Check sheet for the modelled part. Datum: model origin and axes. Units: mm. A direction names the side the tool comes from. Give positions to 0.01 mm unless a question says otherwise; leave off trailing zeros. Loops run counter-clockwise (first coordinate to the right, second up) from the corner with the lowest first, then second, coordinate; pieces in that order, holes last. Notation, with made-up numbers: M 66.5,13 L 79.5,13 A33 cw 79.5,50 Z; hole C -20.5,25.25 d6. An arc over 180 degrees is marked long. Put each result on its own line as item: value. Start each with the question number.
Autodesk Inventor part; units mm, degrees
ref_plane "YZ Plane" through (0, 0, 0) normal (1, 0, 0) x (0, 1, 0)
ref_plane "XZ Plane" through (0, 0, 0) normal (0, 1, 0) x (-1, 0, 0)
ref_plane "XY Plane" through (0, 0, 0) normal (0, 0, 1) x (1, 0, 0)
sketch "Sketch1" plane through (0, 0, 0) normal (0, 0, 1) x (1, 0, 0)
  ellipse E0 centre (87.4656, 123.4744) end of major axis (87.4656, -181.3256) minor radius 228.6
  line L0 (189.0656, 234.7689) -> (176.3656, 234.7689)
  line L1 (176.3656, 234.7689) -> (176.3656, 222.0689)
  line L2 (176.3656, 222.0689) -> (189.0656, 222.0689)
  line L3 (189.0656, 222.0689) -> (189.0656, 234.7689)
  line L4 (-14.1344, 234.7689) -> (-1.4344, 234.7689)
  line L5 (-1.4344, 234.7689) -> (-1.4344, 222.0689)
  line L6 (-1.4344, 222.0689) -> (-14.1344, 222.0689)
  line L7 (-14.1344, 222.0689) -> (-14.1344, 234.7689)
  line L8 (189.0656, -70.0311) -> (176.3656, -70.0311)
  line L9 (176.3656, -70.0311) -> (176.3656, -57.3311)
  line L10 (176.3656, -57.3311) -> (189.0656, -57.3311)
  line L11 (189.0656, -57.3311) -> (189.0656, -70.0311)
  line L12 (-14.1344, -70.0311) -> (-1.4344, -70.0311)
  line L13 (-1.4344, -70.0311) -> (-1.4344, -57.3311)
  line L14 (-1.4344, -57.3311) -> (-14.1344, -57.3311)
  line L15 (-14.1344, -57.3311) -> (-14.1344, -70.0311)
  line L16 (75.0457, -66.5884) -> (75.0457, -5.6676)
  line L17 (75.0457, -5.6676) -> (100.4457, -5.6676)
  line L18 (100.4457, -5.6676) -> (100.4457, -66.5884)
  line L19 (100.4457, -66.5884) -> (75.0457, -66.5884)
  circle A0 centre (87.4656, 239.7517) radius 30.4
  point P0 (0, 0)
  dimension "d2" = 203.2
  dimension "d3" = 12.7
  dimension "d4" = 12.7
  dimension "d5" = 12.7
  dimension "d6" = 12.7
  dimension "d7" = 12.7
extrude "Extrusion1" add sketch "Sketch1" along normal blind 50.8 contours L3 L2 L1 L0 | L4 L5 L6 L7 | L8 L9 L10 L11 | L15 L14 L13 L12
sketch "Sketch2" plane through (0, 0, 50.8) normal (0, 0, 1) x (1, 0, 0)
  line L0 (189.0656, 222.0689) -> (189.0656, 234.7689)
  line L1 (-14.1344, -70.0311) -> (-1.4344, -70.0311)
  line L2 (189.0656, 234.7689) -> (-14.1344, 234.7689)
  line L3 (-14.1344, 234.7689) -> (-14.1344, -70.0311)
  line L4 (-14.1344, -70.0311) -> (189.0656, -70.0311)
  line L5 (189.0656, -70.0311) -> (189.0656, 234.7689)
  point P0 (0, 0)
extrude "Extrusion2" add sketch "Sketch2" along normal blind 12.7
properties part number "base_table"
Q1. Thickness scan on line 1 along Z through (x, y) = (29, 200.5). Record the ranges inside material, lowest first. Write a range as [from, to].
Q2. Access from +Z, -Z, +X, -X, +Y, -Y to the whole of each face (thin tool, end or side, straight path). Record for faces 5 (the face through (-8, 229, 0)), 6 (the face through (183, 222.069, 25)), 7 (the face through (-1.434, -64, 25)).
Q3. Mould release check, pull along X, two halves, no side actions. Record for faces 1 (the face through (-14.134, 83, 55)), 2 (the face through (176.366, 229, 25)), 3 (the face through (189.066, 82, 55)), 4 (the face through (183, 229, 0)): pulls with the +X half, pulls with the -X half, needs draft (parallel to the pull), parting line crosses it, or undercut.
Q4. Section check A-A, the plane z = 14. Record the cut outline in (x, y), then the cut area to 3 significant figures.
Q5. Depth check by flat-ended pin: P1, Ø6, axis at x = 150, y = 1.5, coming from the -Z side. Enter the tip coordinate at first touch or a pass-through.
Q6. Section check B-B, the plane y = 142. Record the cut outline in (x, z), then the cut area to 3 significant figures.
Q7. Section check C-C, the plane x = 15.5. Record the cut outline in (y, z), then the cut area to 3 significant figures.
Found:
1. line 1: z = [50.8, 63.5]
2. face 5: -Z, +X, -X, +Y, -Y
2. face 6: -Z, +X, -X
2. face 7: -Z, +Y, -Y
3. face 1: pulls with the -X half
3. face 2: undercut
3. face 3: pulls with the +X half
3. face 4: needs draft
4. outline: M -14.13,-70.03 L -1.43,-70.03 L -1.43,-57.33 L -14.13,-57.33 Z; M -14.13,222.07 L -1.43,222.07 L -1.43,234.77 L -14.13,234.77 Z; M 176.37,-70.03 L 189.07,-70.03 L 189.07,-57.33 L 176.37,-57.33 Z; M 176.37,222.07 L 189.07,222.07 L 189.07,234.77 L 176.37,234.77 Z
4. area: 645 mm^2
5. P1: stops at z = 50.8
6. outline: M -14.13,50.8 L 189.07,50.8 L 189.07,63.5 L -14.13,63.5 Z
6. area: 2,580 mm^2
7. outline: M -70.03,50.8 L 234.77,50.8 L 234.77,63.5 L -70.03,63.5 Z
7. area: 3,870 mm^2
